Read the model definition and answer for the solid it produces. Units are mm, in the model's axes. A direction names the side the tool comes from. Coordinates: 2 decimals unless noted, no trailing zeros. Loops run counter-clockwise (first coordinate to the right, second up) from the corner with the lowest first, then second, coordinate; pieces in that order, holes last. Notation, with made-up numbers: M 20,29 L 55,29 A17 ccw 55,47 Z; hole C 32.5,75 d8. An arc over 180 degrees is marked long. One line per item, written item: value. Start each with the question number.
1. The part is cut by section D-D (x = -1.4). Write down the section's boundary in (y, z), then the cut area to 3 significant figures.
2. The part is cut by section A-A (x = 1.05). Write down the section's boundary in (y, z), then the cut area to 3 significant figures.
3. Determine the mould class of faces 1 (the face through (-1, 0, 1)), 2 (the face through (1.325, -1.246, -1.277)), 3 (the face through (-2, 8, 0)) for opening direction Y: +Y half, -Y half, draft (parallel to the pull), parting line (faces both ways), or undercut.
4. For faces 4 (the face through (-1.633, 4.302, 0.341)), 5 (the face through (1, -1, 0)), 6 (the face through (-1, -1.5, 0)), determine the directions among +Z, -Z, +X, -X, +Y, -Y from which every point of the face is accessible in a straight line to the end or side of a thin tool.
5. The part is cut by section B-B (z = 1.25). Write down the section's boundary in (x, y).
6. A flat-ended cylindrical pin translates along its axis: pin 1 (2.5 mm diameter, centred on x = -0.52, z = -0.51, fed in from +Y). Find the tip coordinate at first contact, or state that the pin passes through.
7. The part is cut by section C-C (z = -1.4). Write down the section's boundary in (x, y), then the cut area to 3 significant figures.
8. Consider probe 1 along Y at (x, z) = (-1.25, 0.65); probe 2 along Y at (x, z) = (0.95, 0.25); probe 3 along Y at (x, z) = (-1.2, -0.05). Determine where each line is inside the solid, lowest interval first.
```python
from build123d import *

# Parameters (mm, degrees)
SKETCH1_R           = 2.25
BOSS_EXTRUDE1_DEPTH = 8
SKETCH1_3_R         = 1.375
BOSS_EXTRUDE2_DEPTH = 1
SKETCH5_R           = 1.25
BOSS_EXTRUDE3_DEPTH = 1
SKETCH6_R           = 2
BOSS_EXTRUDE4_DEPTH = 0.5
SKETCH12_R          = 1.4
CUT_EXTRUDE1_DEPTH  = 7.5


with BuildPart() as part:
    # Sketch1 → Boss-Extrude1 (new body)
    with BuildSketch(Plane(origin=(0, 0, 0), x_dir=(1, 0, 0), z_dir=(0, 1, 0))):
        with Locations((-0.522013312, 0.511138034)):
            Circle(SKETCH1_R)
    extrude(amount=BOSS_EXTRUDE1_DEPTH)

    # Sketch1<3> → Boss-Extrude2 (add)
    with BuildSketch(Plane(origin=(0, 0, 0), x_dir=(1, 0, 0), z_dir=(0, 1, 0))):
        with Locations((-0.522013312, 0.511138034)):
            Circle(SKETCH1_3_R)
    extrude(amount=BOSS_EXTRUDE2_DEPTH)

    # Sketch5 → Boss-Extrude3 (add)
    with BuildSketch(Plane.XZ):
        with Locations((-0.522013312, -0.511138034)):
            Circle(SKETCH5_R)
    extrude(amount=BOSS_EXTRUDE3_DEPTH)

    # Sketch6 → Boss-Extrude4 (add)
    with BuildSketch(Plane.XZ.offset(1)):
        with Locations((-0.522013312, -0.511138034)):
            Circle(SKETCH6_R)
    extrude(amount=BOSS_EXTRUDE4_DEPTH)

    # Sketch12 → Cut-Extrude1 (cut)
    with BuildSketch(Plane(origin=(0, 8, 0), x_dir=(1, 0, 0), z_dir=(0, 1, 0))):
        with Locations((-0.522013312, 0.511138034)):
            Circle(SKETCH12_R)
    extrude(amount=-CUT_EXTRUDE1_DEPTH, mode=Mode.SUBTRACT)


solid = part.part
```
Answer block:
1. outline: M -1.5,-2.31 L -1,-2.31 L -1,-1.4 L 0,-1.4 L 0,-2.58 L 8,-2.58 L 8,-1.6 L 0.5,-1.6 L 0.5,0.58 L 8,0.58 L 8,1.56 L 0,1.56 L 0,0.38 L -1,0.38 L -1,1.29 L -1.5,1.29 Z
1. area: 20.4 mm2
2. outline: M -1.5,-1.75 L -1,-1.75 L -1,0.73 L -1.5,0.73 Z; M 0,-2.12 L 8,-2.12 L 8,1.1 L 0,1.1 Z
2. area: 27.0 mm2
3. face 1: undercut
3. face 2: draft
3. face 3: +Y half
4. face 4: +Y
4. face 5: none
4. face 6: +Z, -Z, +X, -X, -Y
5. outline: M -1.92,0 L 0.88,0 L 0.88,8 L -1.92,8 Z; M -1.47,-1.5 L 0.43,-1.5 L 0.43,-1 L -1.47,-1 Z
6. pin 1: stops at y = 0.5
7. outline: M -2.59,0 L -1.4,0 L -1.4,-1 L -2.31,-1 L -2.31,-1.5 L 1.27,-1.5 L 1.27,-1 L 0.36,-1 L 0.36,0 L 1.54,0 L 1.54,8 L 0.56,8 L 0.56,0.5 L -1.6,0.5 L -1.6,8 L -2.59,8 Z
7. area: 20.4 mm2
8. probe 1: y = -1.5 to -1, 0 to 0.5
8. probe 2: y = -1.5 to -1, 0 to 8
8. probe 3: y = -1.5 to 0.5
